For this review, use the dimensioned drawing (mm, ordinates from the lowest corner) and the shaded views. A direction names the side the tool comes from. Round coordinates to 2 decimals unless told otherwise and drop trailing zeros. Order: outer loops, then holes, each group sorted by start corner. A loop starts at its lowest first (then second) coordinate and runs counter-clockwise, first axis right, second up. Notation, with made-up numbers: (67.25, -23) - (80.25, -23) arc R18 cw to (80.25, -12) - close; hole circle Ø8 at (26, -34). An arc over 180 degrees is marked (long way). Write item = value, one per line.
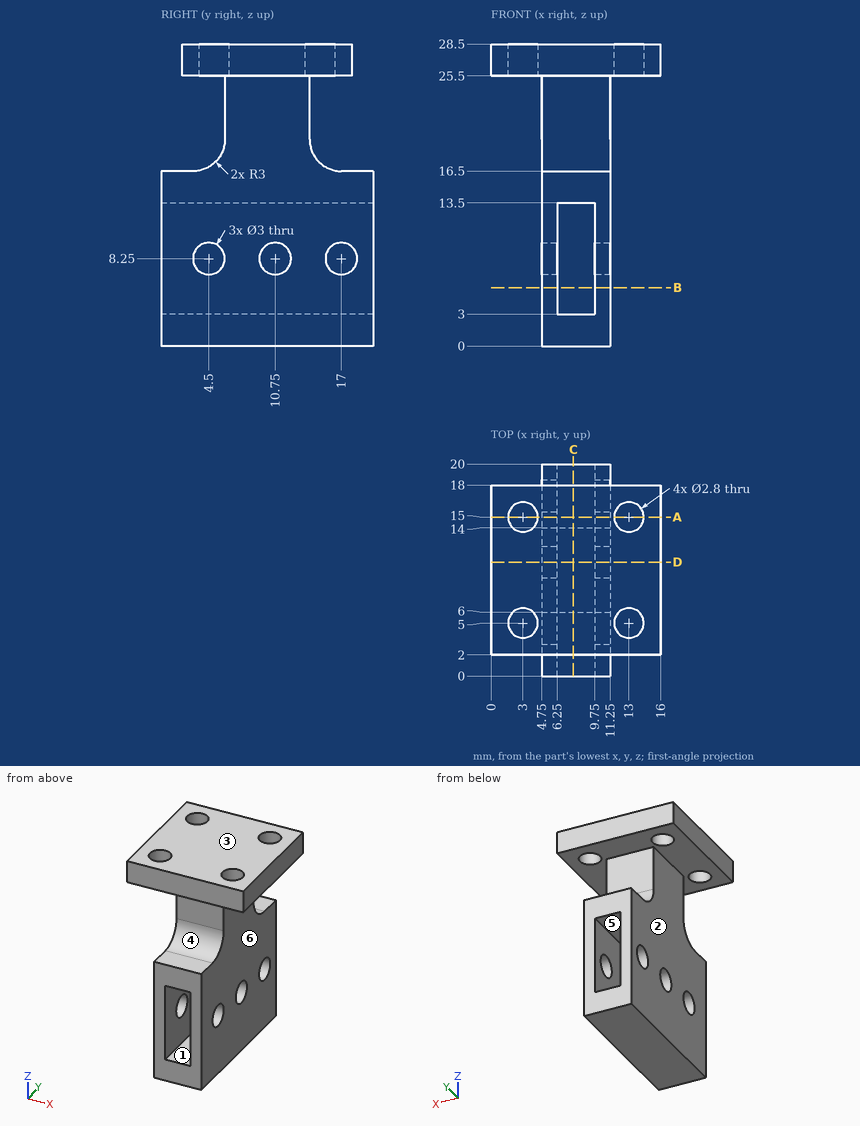
1) We need section D-D on y = 10.75. Write out the cut boundary in (x, z), and give its area (3 significant figures).
Findings:
outline = (0, 25.5) - (4.75, 25.5) - (4.75, 9.75) - (6.25, 9.75) - (6.25, 13.5) - (9.75, 13.5) - (9.75, 9.75) - (11.25, 9.75) - (11.25, 25.5) - (16, 25.5) - (16, 28.5) - (0, 28.5) - close; (4.75, 0) - (11.25, 0) - (11.25, 6.75) - (9.75, 6.75) - (9.75, 3) - (6.25, 3) - (6.25, 6.75) - (4.75, 6.75) - close
area = 168 mm^2
2) The part is to be moulded in two halves that separate along Z. For the marked faces 1, 2 and 3, say which applies: released by +Z, released by -Z, zero draft, split by the parting line, or undercut.
Findings:
face_1 = undercut
face_2 = zero draft
face_3 = released by +Z
3) We need section C-C on x = 7.75. Write out the cut boundary in (y, z), and give its area (3 significant figures).
Findings:
outline = (0, 0) - (20, 0) - (20, 3) - (0, 3) - close; (0, 13.5) - (20, 13.5) - (20, 16.5) - (17, 16.5) arc R3 cw to (14, 19.5) - (14, 25.5) - (18, 25.5) - (18, 28.5) - (2, 28.5) - (2, 25.5) - (6, 25.5) - (6, 19.5) arc R3 cw to (3, 16.5) - (0, 16.5) - close
area = 244 mm^2
4) To check wall thickness, follow L1, parallel to Y at x = 3, z = 27.8; L2, parallel to Y at x = 10.9, z = 8.25; L3, parallel to X at y = 3, z = 11.75. State the ranges of each line that lie inside material, in increasing order. Write a range as from..to.
Findings:
L1 = 2..3.6, 6.4..13.6, 16.4..18
L2 = 0..3, 6..9.25, 12.25..15.5, 18.5..20
L3 = 4.75..6.25, 9.75..11.25
5) We need section B-B on z = 5.5. Write out the cut boundary in (x, y), and give its area (3 significant figures).
Findings:
outline = (4.75, 0) - (6.25, 0) - (6.25, 20) - (4.75, 20) - close; (9.75, 0) - (11.25, 0) - (11.25, 20) - (9.75, 20) - close
area = 60.0 mm^2
6) For the marked faces 4, 5 and 6, list the 3-axis set-ups (+Z, -Z, +X, -X, +Y, -Y) from which the entire face can be reached by the end or side of a thin tool; tool diameter is ignored.
Findings:
face_4 = +X, -X, -Y
face_5 = +Y, -Y
face_6 = -Z, +X, +Y, -Y
7) Clearance check with flat-ended pins moving along their axes: pin 1 Ø5 at (y, z) = (17, 8.25) entering from -X; pin 2 Ø5 at (x, z) = (8.5, 23.5) entering from +Y; pin 3 Ø1.8 at (x, z) = (7.5, 23) entering from -Y; pin 4 Ø2.5 at (y, z) = (4.5, 8.25) entering from +X. State where each tip first meets the part, or that it passes through.
Findings:
pin_1 = 4.75
pin_2 = 18
pin_3 = 6
pin_4 = through
8) We need section A-A on y = 15. Write out the cut boundary in (x, z).
Findings:
outline = (0, 25.5) - (1.6, 25.5) - (1.6, 28.5) - (0, 28.5) - close; (4.4, 25.5) - (11.6, 25.5) - (11.6, 28.5) - (4.4, 28.5) - close; (4.75, 0) - (11.25, 0) - (11.25, 17.26) - (4.75, 17.26) - close; (14.4, 25.5) - (16, 25.5) - (16, 28.5) - (14.4, 28.5) - close; hole (6.25, 3) - (9.75, 3) - (9.75, 13.5) - (6.25, 13.5) - close
